from build123d import *

# Parameters (mm, degrees)
SKETCH1_W               = 7.47
SKETCH1_H               = 4.93
BOSS_EXTRUDE1_DEPTH     = 0.8
BOSS_EXTRUDE2_DEPTH     = 1.7
SKETCH3_R               = 1.609625666
BOSS_EXTRUDE3_DEPTH     = 1.8
FILLET1_R               = 0.9
SKETCH4_W               = 0.6
SKETCH4_H               = 2
CUT_EXTRUDE1_DEPTH      = 1.8
CUT_EXTRUDE2_DEPTH      = 10.129392113
SKETCH6_W               = 0.55
SKETCH6_H               = 0.3
CUT_EXTRUDE3_DEPTH      = 0.05
LPATTERN1_COUNT         = 5
LPATTERN1_PITCH         = 1.27
MIRROR1_COPY_1_DEPTH    = 10.129392113
MIRROR1_COPY_2_DEPTH    = 10.129392113
MIRROR1_COPY_3_DEPTH    = 10.129392113
MIRROR1_COPY_4_DEPTH    = 10.129392113
MIRROR1_COPY_5_SKETCH_W = 0.55
MIRROR1_COPY_5_SKETCH_H = 0.3
MIRROR1_COPY_5_DEPTH    = 0.05
MIRROR1_COPY_6_SKETCH_W = 0.55
MIRROR1_COPY_6_SKETCH_H = 0.3
MIRROR1_COPY_6_DEPTH    = 0.05
MIRROR1_COPY_7_SKETCH_W = 0.55
MIRROR1_COPY_7_SKETCH_H = 0.3
MIRROR1_COPY_7_DEPTH    = 0.05
MIRROR1_COPY_8_SKETCH_W = 0.55
MIRROR1_COPY_8_SKETCH_H = 0.3
MIRROR1_COPY_8_DEPTH    = 0.05


with BuildPart() as part:
    # Sketch1 → Boss-Extrude1 (new body)
    with BuildSketch(Plane.XY):
        with Locations((3.735, 2.465)):
            Rectangle(SKETCH1_W, SKETCH1_H)
    extrude(amount=BOSS_EXTRUDE1_DEPTH)

    # Sketch2 → Boss-Extrude2 (add)
    with BuildSketch(Plane.XY.offset(0.8)):
        Polygon((2.939618782, 3.62939168), (2.939618782, 1.30060832), (2.32, 1.115), (2.32, 0.815), (6.52, 0.815), (6.52, 4.115), (2.32, 4.115), (2.32, 3.815), align=None)
    extrude(amount=BOSS_EXTRUDE2_DEPTH)

    # Sketch3 → Boss-Extrude3 (add)
    with BuildSketch(Plane.XY.offset(0.8)):
        with Locations(Location((1.729625666, 2.465, 0), (0, 0, 68.482991379))):
            Circle(SKETCH3_R)
    extrude(amount=BOSS_EXTRUDE3_DEPTH)

    # Fillet1
    # the kernel refuses this fillet: 0.9 mm, written as the material it takes off along each edge
    with BuildSketch(Plane(origin=(1.729625666, 2.465, 2.6), x_dir=(0.3667774110162909, 0.9303087287391142, 0), z_dir=(0.9303087287391142, -0.3667774110162909, 0))) as fillet1_piece_1_section:
        with BuildLine():
            CenterArc((1.609625666 - FILLET1_R, -FILLET1_R), FILLET1_R, 0, 90)
            Line((1.609625666 - FILLET1_R, 0), (1.609625666, 0))
            Line((1.609625666, 0), (1.609625666, -FILLET1_R))
        make_face()
    fillet1_piece_1 = revolve(axis=Axis((1.729625666, 2.465, 2.6), (0, 0, 1)), mode=Mode.PRIVATE)
    fillet1_piece_1 = split(fillet1_piece_1, bisect_by=Plane(origin=(2.32, 3.98462035, 2.239901454), z_dir=(-1, 0, 0)), keep=Keep.TOP, mode=Mode.PRIVATE)
    add(fillet1_piece_1, mode=Mode.SUBTRACT)
    with BuildSketch(Plane(origin=(1.729625666, 2.465, 2.6), x_dir=(0.3667774110162909, 0.9303087287391142, 0), z_dir=(0.9303087287391142, -0.3667774110162909, 0))) as fillet1_piece_2_section:
        with BuildLine():
            CenterArc((1.609625666 - FILLET1_R, -FILLET1_R), FILLET1_R, 0, 90)
            Line((1.609625666 - FILLET1_R, 0), (1.609625666, 0))
            Line((1.609625666, 0), (1.609625666, -FILLET1_R))
        make_face()
    fillet1_piece_2 = revolve(axis=Axis((1.729625666, 2.465, 2.6), (0, 0, 1)), mode=Mode.PRIVATE)
    fillet1_piece_2 = split(fillet1_piece_2, bisect_by=Plane(origin=(2.8939742, 1.286935374, 1.864268615), z_dir=(-0.28695452749278183, 0.9579442046128753, 0)), keep=Keep.TOP, mode=Mode.PRIVATE)
    fillet1_piece_2 = split(fillet1_piece_2, bisect_by=Plane(origin=(2.939618782, 1.348625417, 1.864268615), z_dir=(-1, 0, 0)), keep=Keep.TOP, mode=Mode.PRIVATE)
    fillet1_piece_2 = split(fillet1_piece_2, bisect_by=Plane(origin=(3.507726639, 3.459213583, 1.864268615), z_dir=(-0.28695452749278183, -0.9579442046128753, 0)), keep=Keep.TOP, mode=Mode.PRIVATE)
    add(fillet1_piece_2, mode=Mode.SUBTRACT)
    with BuildSketch(Plane(origin=(1.729625666, 2.465, 2.6), x_dir=(0.3667774110162909, 0.9303087287391142, 0), z_dir=(0.9303087287391142, -0.3667774110162909, 0))) as fillet1_piece_3_section:
        with BuildLine():
            CenterArc((1.609625666 - FILLET1_R, -FILLET1_R), FILLET1_R, 0, 90)
            Line((1.609625666 - FILLET1_R, 0), (1.609625666, 0))
            Line((1.609625666, 0), (1.609625666, -FILLET1_R))
        make_face()
    fillet1_piece_3 = revolve(axis=Axis((1.729625666, 2.465, 2.6), (0, 0, 1)), mode=Mode.PRIVATE)
    fillet1_piece_3 = split(fillet1_piece_3, bisect_by=Plane(origin=(2.494750344, 3.818777252, 2.5), z_dir=(0, 0, 1)), keep=Keep.TOP, mode=Mode.PRIVATE)
    add(fillet1_piece_3, mode=Mode.SUBTRACT)

    # Sketch4 → Cut-Extrude1 (cut)
    with BuildSketch(Plane.XY.offset(2.5)):
        with Locations((5.5, 2.465)):
            Rectangle(SKETCH4_W, SKETCH4_H)
    extrude(amount=-CUT_EXTRUDE1_DEPTH, mode=Mode.SUBTRACT)

    # Sketch5 → Cut-Extrude2 (cut, through all)
    with BuildSketch(Plane.XY.offset(0.8)):
        with BuildLine():
            Line((1.58, 4.93), (2.08, 4.93))
            ThreePointArc((2.08, 4.93), (1.83, 4.68), (1.58, 4.93))
        make_face()
    cut_extrude2 = extrude(amount=-CUT_EXTRUDE2_DEPTH, mode=Mode.SUBTRACT)

    # Sketch6 → Cut-Extrude3 (cut)
    with BuildSketch(Plane.XY.offset(0.8)):
        with Locations((1.83, 4.78)):
            Rectangle(SKETCH6_W, SKETCH6_H)
    cut_extrude3 = extrude(amount=-CUT_EXTRUDE3_DEPTH, mode=Mode.SUBTRACT)

    # LPattern1: Cut-Extrude2, Cut-Extrude3 ×5
    with Locations(*[(i * LPATTERN1_PITCH, 0, 0) for i in range(1, LPATTERN1_COUNT)]):
        add(cut_extrude2, mode=Mode.SUBTRACT)
        add(cut_extrude3, mode=Mode.SUBTRACT)

    # Mirror1: Cut-Extrude2, Cut-Extrude3 across plane
    add(cut_extrude2.mirror(Plane.ZX.offset(2.465)), mode=Mode.SUBTRACT)
    add(cut_extrude3.mirror(Plane.ZX.offset(2.465)), mode=Mode.SUBTRACT)

    # Mirror1 copy 1 sketch → Mirror1 copy 1 (cut, through all)
    with BuildSketch(Plane(origin=(1.27, 4.93, 0.8), x_dir=(1, 0, 0), z_dir=(0, 0, 1))):
        with BuildLine():
            Line((1.58, -4.93), (2.08, -4.93))
            ThreePointArc((2.08, -4.93), (1.83, -4.68), (1.58, -4.93))
        make_face()
    extrude(amount=-MIRROR1_COPY_1_DEPTH, mode=Mode.SUBTRACT)

    # Mirror1 copy 2 sketch → Mirror1 copy 2 (cut, through all)
    with BuildSketch(Plane(origin=(2.54, 4.93, 0.8), x_dir=(1, 0, 0), z_dir=(0, 0, 1))):
        with BuildLine():
            Line((1.58, -4.93), (2.08, -4.93))
            ThreePointArc((2.08, -4.93), (1.83, -4.68), (1.58, -4.93))
        make_face()
    extrude(amount=-MIRROR1_COPY_2_DEPTH, mode=Mode.SUBTRACT)

    # Mirror1 copy 3 sketch → Mirror1 copy 3 (cut, through all)
    with BuildSketch(Plane(origin=(3.81, 4.93, 0.8), x_dir=(1, 0, 0), z_dir=(0, 0, 1))):
        with BuildLine():
            Line((1.58, -4.93), (2.08, -4.93))
            ThreePointArc((2.08, -4.93), (1.83, -4.68), (1.58, -4.93))
        make_face()
    extrude(amount=-MIRROR1_COPY_3_DEPTH, mode=Mode.SUBTRACT)

    # Mirror1 copy 4 sketch → Mirror1 copy 4 (cut, through all)
    with BuildSketch(Plane(origin=(5.08, 4.93, 0.8), x_dir=(1, 0, 0), z_dir=(0, 0, 1))):
        with BuildLine():
            Line((1.58, -4.93), (2.08, -4.93))
            ThreePointArc((2.08, -4.93), (1.83, -4.68), (1.58, -4.93))
        make_face()
    extrude(amount=-MIRROR1_COPY_4_DEPTH, mode=Mode.SUBTRACT)

    # Mirror1 copy 5 sketch → Mirror1 copy 5 (cut)
    with BuildSketch(Plane(origin=(1.27, 4.93, 0.8), x_dir=(1, 0, 0), z_dir=(0, 0, 1))):
        with Locations((1.83, -4.78)):
            Rectangle(MIRROR1_COPY_5_SKETCH_W, MIRROR1_COPY_5_SKETCH_H)
    extrude(amount=-MIRROR1_COPY_5_DEPTH, mode=Mode.SUBTRACT)

    # Mirror1 copy 6 sketch → Mirror1 copy 6 (cut)
    with BuildSketch(Plane(origin=(2.54, 4.93, 0.8), x_dir=(1, 0, 0), z_dir=(0, 0, 1))):
        with Locations((1.83, -4.78)):
            Rectangle(MIRROR1_COPY_6_SKETCH_W, MIRROR1_COPY_6_SKETCH_H)
    extrude(amount=-MIRROR1_COPY_6_DEPTH, mode=Mode.SUBTRACT)

    # Mirror1 copy 7 sketch → Mirror1 copy 7 (cut)
    with BuildSketch(Plane(origin=(3.81, 4.93, 0.8), x_dir=(1, 0, 0), z_dir=(0, 0, 1))):
        with Locations((1.83, -4.78)):
            Rectangle(MIRROR1_COPY_7_SKETCH_W, MIRROR1_COPY_7_SKETCH_H)
    extrude(amount=-MIRROR1_COPY_7_DEPTH, mode=Mode.SUBTRACT)

    # Mirror1 copy 8 sketch → Mirror1 copy 8 (cut)
    with BuildSketch(Plane(origin=(5.08, 4.93, 0.8), x_dir=(1, 0, 0), z_dir=(0, 0, 1))):
        with Locations((1.83, -4.78)):
            Rectangle(MIRROR1_COPY_8_SKETCH_W, MIRROR1_COPY_8_SKETCH_H)
    extrude(amount=-MIRROR1_COPY_8_DEPTH, mode=Mode.SUBTRACT)


solid = part.part
Geometry: final body of the model. Coordinates: model frame, mm. A direction names the side the tool comes from. Give positions to 0.01 mm unless a question says otherwise; leave off trailing zeros. Write each loop counter-clockwise with the first axis right and the second up, starting at its lowest first coordinate (ties: lowest second). Pieces come first, ordered by that corner, then holes. Notation, with made-up numbers: (-12, 76.25) -> (41, 76.25) arc R4 ccw to (41, 80.25) -> close; hole circle Ø5 at (85, -16.5). An arc over 180 degrees is marked (long way). Answer in a Markdown table with one row per item.
(1) Set-up query: faces 1 (the flat face through (6.52, 2, 2)), 2 (the flat face through (2, 2, 2.6)), 3 (the flat face through (5.2, 2, 2)). Return all of +Z, -Z, +X, -X, +Y, -Y with unobstructed straight access to the full face (end or side cutting, diameter ignored); none if empty.
Answers below:
| item | result |
|---|---|
| face 1 | +Z, +X, +Y, -Y |
| face 2 | +Z, +X, -X, +Y, -Y |
| face 3 | +Z |
(2) Ray query, line 1 along Y through (x, z) = (5.5, 1.5) (3 decimals); line 2 along Y through (x, z) = (2.5, 2.45) (3 decimals); line 3 along Z through (x, y) = (6.25, 1.5). Return the intervals inside material, ascending. Write a range as [from, to].
Answers below:
| item | result |
|---|---|
| line 1 | [0.815, 1.465], [3.465, 4.115] |
| line 2 | [0.815, 1.169], [1.536, 3.394], [3.761, 4.115] |
| line 3 | [0, 2.5] |
(3) Section query C-C on x = 3.5. Return loops of the section in (y, z) (3 decimals).
Answers below:
| item | result |
|---|---|
| outline | (0, 0) -> (4.93, 0) -> (4.93, 0.8) -> (4.115, 0.8) -> (4.115, 2.5) -> (0.815, 2.5) -> (0.815, 0.8) -> (0, 0.8) -> close |
(4) Section query D-D on x = 5.64. Return loops of the section in (y, z) (3 decimals), then the cut area to 3 significant figures.
Answers below:
| item | result |
|---|---|
| outline | (0.25, 0) -> (4.68, 0) -> (4.68, 0.75) -> (4.63, 0.75) -> (4.63, 0.8) -> (4.115, 0.8) -> (4.115, 2.5) -> (3.465, 2.5) -> (3.465, 0.7) -> (1.465, 0.7) -> (1.465, 2.5) -> (0.815, 2.5) -> (0.815, 0.8) -> (0.3, 0.8) -> (0.3, 0.75) -> (0.25, 0.75) -> close |
| area | 5.55 mm^2 |
(5) Pin query (flat end, axial travel): pin 1 (1.4 mm diameter, centred on y = 2.5, z = 1, fed in from +X); pin 2 (2.5 mm diameter, centred on x = 4, y = 3.5, fed in from +Z). Return the tip coordinate at first contact, or that it passes through.
Answers below:
| item | result |
|---|---|
| pin 1 | x = 7.47 |
| pin 2 | z = 2.5 |
(6) Section query B-B on z = 1.3. Return loops of the section in (x, y) (3 decimals), then the cut area to 3 significant figures.
Answers below:
| item | result |
|---|---|
| outline | (2.32, 0.815) -> (6.52, 0.815) -> (6.52, 4.115) -> (2.32, 4.115) -> (2.32, 3.962) arc R1.61 ccw (long way) to (2.32, 0.968) -> close; hole (2.793, 1.257) -> (2.94, 1.301) -> (2.94, 1.403) arc R1.61 cw to start; hole (2.793, 3.673) arc R1.61 cw to (2.94, 3.527) -> (2.94, 3.629) -> close; hole (5.2, 1.465) -> (5.8, 1.465) -> (5.8, 3.465) -> (5.2, 3.465) -> close |
| area | 18.6 mm^2 |
(7) Section query A-A on x = 4.37. Return loops of the section in (y, z) (3 decimals).
Answers below:
| item | result |
|---|---|
| outline | (0.25, 0) -> (4.68, 0) -> (4.68, 0.75) -> (4.63, 0.75) -> (4.63, 0.8) -> (4.115, 0.8) -> (4.115, 2.5) -> (0.815, 2.5) -> (0.815, 0.8) -> (0.3, 0.8) -> (0.3, 0.75) -> (0.25, 0.75) -> close |
(8) Draft query along Y for faces 4 (the flat face through (5.8, 2, 2)), 5 (the flat face through (4, 4.115, 2)), 6 (the flat face through (4, 2, 2.5)), 7 (the flat face through (4, 0.815, 2)). Return one class per face: +Y half, -Y half, draft (parallel to the pull), parting line (faces both ways), or undercut.
Answers below:
| item | result |
|---|---|
| face 4 | undercut |
| face 5 | +Y half |
| face 6 | draft |
| face 7 | -Y half |
